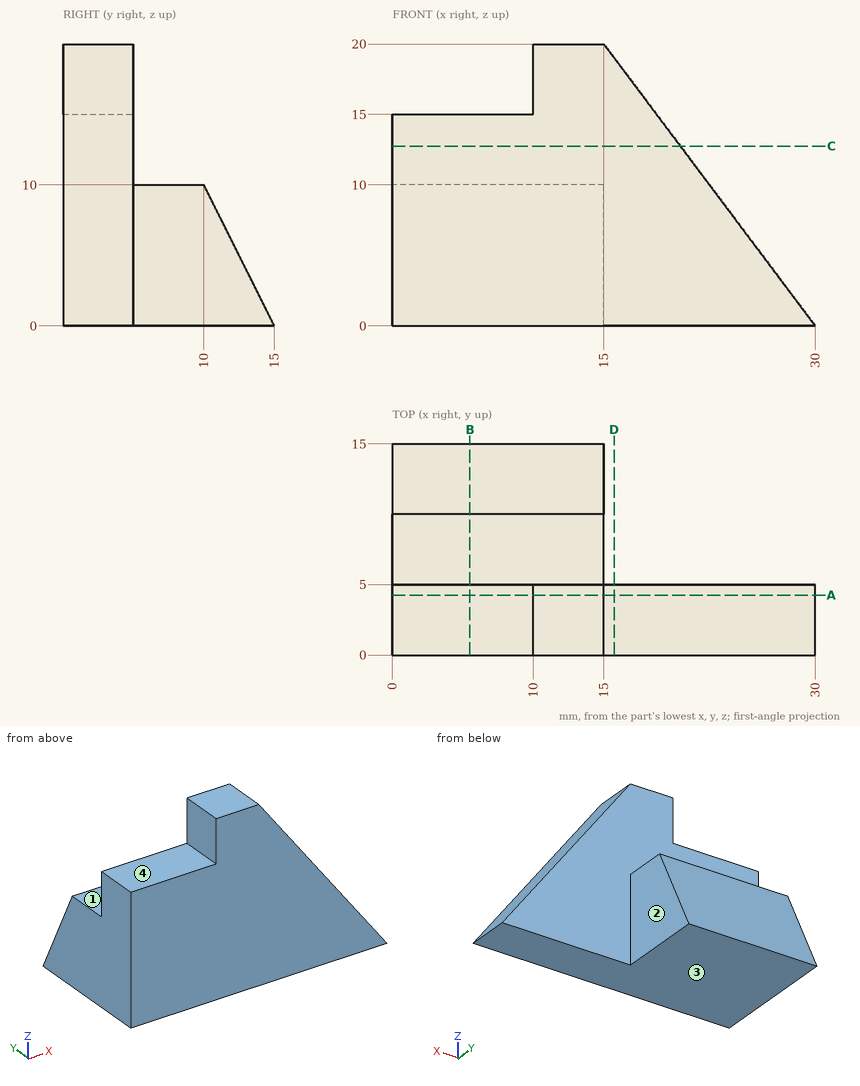
For this review, use the dimensioned drawing (mm, ordinates from the lowest corner) and the shaded views. A direction names the side the tool comes from. Coordinates: 2 decimals unless noted, no trailing zeros. Loops run counter-clockwise (first coordinate to the right, second up) from the corner with the lowest first, then second, coordinate; pieces in that order, holes last.
1. Add section B-B, the plane x = 5.5. Give the boundary of the cut face in (y, z), then the cut area to 3 significant figures.
2. For the marked faces 1, 2, 3 and 4, list the 3-axis set-ups (+Z, -Z, +X, -X, +Y, -Y) from which the entire face can be reached by the end or side of a thin tool; tool diameter is ignored.
3. Add section C-C, the plane z = 12.75. Give the boundary of the cut face in (x, y), then the cut area to 3 significant figures.
4. Add section D-D, the plane x = 15.75. Give the boundary of the cut face in (y, z).
5. Add section A-A, the plane y = 4.25. Give the boundary of the cut face in (x, z).
6. Insertion check: P1, Ø1.5, axis at x = 6.5, y = 1.5, coming from the +Z side; P2, Ø8, axis at x = 12.5, y = 10, coming from the +Z side; P3, Ø2.5, axis at y = 3.5, z = 17, coming from the -X side. Each pin has a flat end and moves straight along its axis. Give the tip position at first contact, or say it passes through.
7. For line 1 (X direction, y = 8.25, z = 9.25); line 2 (Z direction, x = 5.5, y = 12.5); line 3 (Z direction, x = 6.5, y = 9.5), list the stretches that pass through material, from the lowest coordinate up.
Result:
1. outline: (0, 0) - (15, 0) - (10, 10) - (5, 10) - (5, 15) - (0, 15) - close
1. area: 150 mm2
2. face 1: +Z, +X, -X, +Y
2. face 2: +Z, -Z, +X, +Y
2. face 3: -Z, +X, -X, +Y, -Y
2. face 4: +Z, -X, +Y, -Y
3. outline: (0, 0) - (20.44, 0) - (20.44, 5) - (0, 5) - close
3. area: 102 mm2
4. outline: (0, 0) - (5, 0) - (5, 19) - (0, 19) - close
5. outline: (0, 0) - (30, 0) - (15, 20) - (10, 20) - (10, 15) - (0, 15) - close
6. P1: stops at z = 15
6. P2: stops at z = 10
6. P3: stops at x = 10
7. line 1: x = 0 to 15
7. line 2: z = 0 to 5
7. line 3: z = 0 to 10
